CAD build for the part. Positions are in the model's coordinates, mm. A direction names the side the tool comes from. Coordinates: 2 decimals unless noted, no trailing zeros. Write each loop counter-clockwise with the first axis right and the second up, starting at its lowest first coordinate (ties: lowest second). Pieces come first, ordered by that corner, then holes. Notation, with made-up numbers: (48.5, 50.5) - (80.5, 50.5) arc R20 cw to (80.5, 76.5) - close; hole circle Ø10 at (-35.75, -1.5). An arc over 180 degrees is marked (long way). Answer in a Markdown table with one row per item. Add a question column.
Q1. Pin check, flat tips, straight feed: pin 1 (3 mm diameter, centred on y = 6, z = 0, fed in from -X); pin 2 (8 mm diameter, centred on x = 9, y = -2, fed in from -Z); pin 3 (1 mm diameter, centred on x = -5.66, y = 5.66, fed in from +Z); pin 4 (1.5 mm diameter, centred on x = 5.66, y = 5.66, fed in from +Z). Stop position of each tip, or through.
Q2. Band-saw the part on A-A (x = 0). State how many separate pieces and enclosed holes the cut face has, and give its area (3 significant figures).
Q3. Drill centre lines: line 1 along Y through (x, z) = (0, 1.55); line 2 along Y through (x, z) = (0, 3.65); line 3 along Y through (x, z) = (5.5, 0.4). Where is each one in solid material? Low to high. Write a range as from..to.
Q4. 3-axis set-ups, long thin cutter, end or side, ignore diameter. For faces 4 (the flat face through (1, -1, 5)), 5 (the flat face through (1.15, 0.04, 2)), 6 (the flat face through (0, -5, 2)): which of +Z, -Z, +X, -X, +Y, -Y reach the whole face in a straight line?
Q5. Band-saw the part on C-C (x = 6). List the corners of the cut face in (y, z), and give its area (3 significant figures).
Q6. Two-plate mould, pull along X, no slides. Class faces 1 (the cylindrical face through (-5.796, 5.031, 0.986)), 2 (the cylindrical face through (-0.867, -3.905, 3.479)), 3 (the flat face through (0, -5, 0)): +X half, -X half, draft (parallel to the pull), parting line (faces both ways), or undercut.
```python
from build123d import *

# Parameters (mm, degrees)
SKETCH1_R           = 11.747376147
SKETCH1_R_2         = 2.669858215
SKETCH1_R_3         = 0.640765972
BOSS_EXTRUDE1_DEPTH = 2
SKETCH2_R           = 4
SKETCH2_R_2         = 1
BOSS_EXTRUDE2_DEPTH = 3
SKETCH3_R           = 4
SKETCH3_R_2         = 2.669858215
BOSS_EXTRUDE3_DEPTH = 1
CHAMFER1_SIZE       = 0.6


with BuildPart() as part:
    # Sketch1 → Boss-Extrude1 (new body)
    with BuildSketch(Plane.XY):
        Circle(SKETCH1_R)
        Circle(SKETCH1_R_2, mode=Mode.SUBTRACT)
        with Locations((0, 8)):
            Circle(SKETCH1_R_3, mode=Mode.SUBTRACT)
        with Locations((5.656854249, 5.656854249)):
            Circle(SKETCH1_R_3, mode=Mode.SUBTRACT)
        with Locations((8, 0)):
            Circle(SKETCH1_R_3, mode=Mode.SUBTRACT)
        with Locations((5.656854249, -5.656854249)):
            Circle(SKETCH1_R_3, mode=Mode.SUBTRACT)
        with Locations((0, -8)):
            Circle(SKETCH1_R_3, mode=Mode.SUBTRACT)
        with Locations((-5.656854249, -5.656854249)):
            Circle(SKETCH1_R_3, mode=Mode.SUBTRACT)
        with Locations((-8, 0)):
            Circle(SKETCH1_R_3, mode=Mode.SUBTRACT)
        with Locations((-5.656854249, 5.656854249)):
            Circle(SKETCH1_R_3, mode=Mode.SUBTRACT)
    extrude(amount=BOSS_EXTRUDE1_DEPTH)

    # Sketch2 → Boss-Extrude2 (add)
    with BuildSketch(Plane.XY.offset(2)):
        Circle(SKETCH2_R)
        Circle(SKETCH2_R_2, mode=Mode.SUBTRACT)
    extrude(amount=BOSS_EXTRUDE2_DEPTH)

    # Sketch3 → Boss-Extrude3 (add)
    with BuildSketch(Plane(origin=(0, 0, 0), x_dir=(-1, 0, 0), z_dir=(0, 0, -1))):
        Circle(SKETCH3_R)
        Circle(SKETCH3_R_2, mode=Mode.SUBTRACT)
    extrude(amount=BOSS_EXTRUDE3_DEPTH)

    # Chamfer1
    chamfer1_edges = [part.edges().sort_by_distance(p)[0] for p in [
        (4, 0, -1),
    ]]
    chamfer(chamfer1_edges, length=CHAMFER1_SIZE)


solid = part.part
```
Checked values:
| question | item | result |
|---|---|---|
| 1 | pin 1 | stops at x = -10.85 |
| 1 | pin 2 | stops at z = 0 |
| 1 | pin 3 | passes through |
| 1 | pin 4 | stops at z = 2 |
| 2 | separate pieces | 4 |
| 2 | enclosed holes | 0 |
| 2 | area | 51.5 mm² |
| 3 | line 1 | y = -11.75..-8.64, -7.36..-2.67, 2.67..7.36, 8.64..11.75 |
| 3 | line 2 | y = -4..-1, 1..4 |
| 3 | line 3 | y = -10.38..-6.28, -5.04..5.04, 6.28..10.38 |
| 4 | face 4 | +Z, +X, -X, +Y, -Y |
| 4 | face 5 | -Z |
| 4 | face 6 | +Z |
| 5 | outline | (-10.1, 0) - (-6.2, 0) - (-6.2, 2) - (-10.1, 2) - close; (-5.12, 0) - (5.12, 0) - (5.12, 2) - (-5.12, 2) - close; (6.2, 0) - (10.1, 0) - (10.1, 2) - (6.2, 2) - close |
| 5 | area | 36.1 mm² |
| 6 | face 1 | undercut |
| 6 | face 2 | parting line |
| 6 | face 3 | draft |
